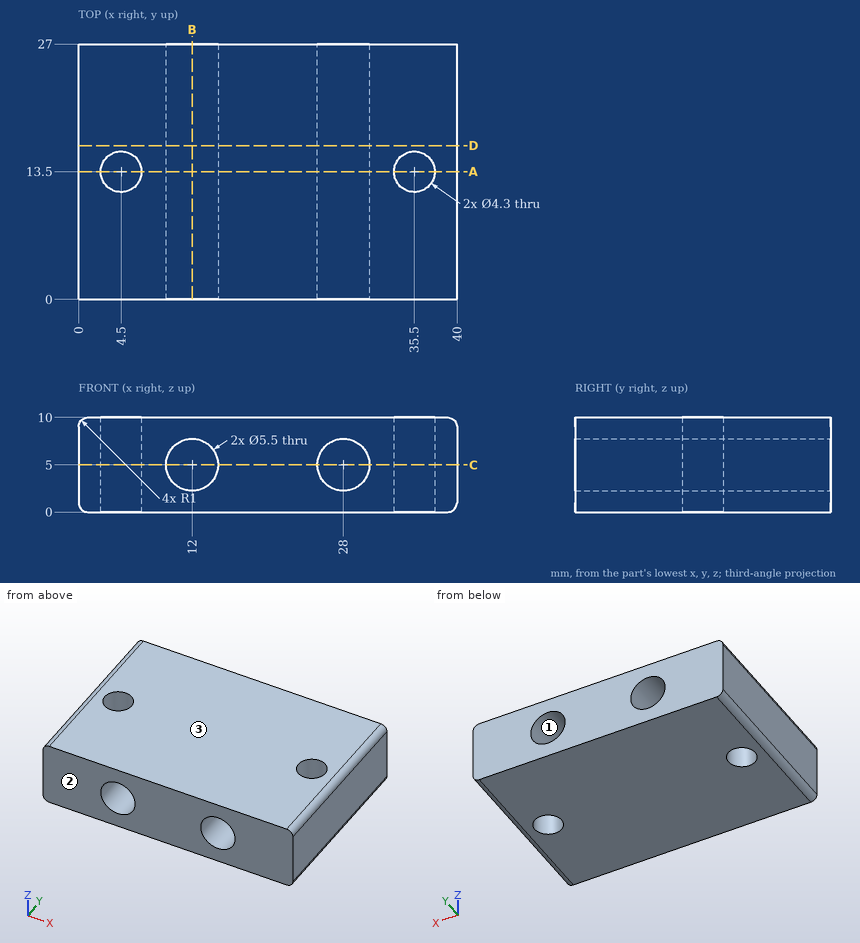
The figure shows three views and two pictorial views of one solid part (mm, origin at its lowest corner). Answer the questions. Coordinates: 2 decimals unless noted, no trailing zeros. Loops run counter-clockwise (first coordinate to the right, second up) from the corner with the lowest first, then second, coordinate; pieces in that order, holes last. Notation, with made-up numbers: M 83,24.5 L 87,24.5 A28 ccw 87,46.5 Z; hole C 84.5,44.5 d7. An arc over 180 degrees is marked long. Use CSV: the item, a comma, the result in double quotes. Start each with the question number.
(1) Find section C-C, the plane z = 5. Give the vertices of the cut face in (x, y).
(2) For a pull along Z with two mould halves and no side action, classify the marked faces 1, 2 and 3 as +Z half, -Z half, draft (parallel to the pull), parting line (faces both ways), or undercut.
(3) Find section A-A, the plane y = 13.5. Give the vertices of the cut face in (x, z).
(4) Find section B-B, the plane x = 12. Give the vertices of the cut face in (y, z), then the cut area to 4 significant figures.
(5) Consider line 1 (X direction, y = 6.75, z = 5); line 2 (Z direction, x = 28, y = 12.5); line 3 (Y direction, x = 4.5, z = 6.5). Determine where each line is inside the solid, lowest interval first.
(6) Find section D-D, the plane y = 16.25. Give the vertices of the cut face in (x, z).
Recorded:
1,outline,"M 0,0 L 9.25,0 L 9.25,27 L 0,27 Z; M 14.75,0 L 25.25,0 L 25.25,27 L 14.75,27 Z; M 30.75,0 L 40,0 L 40,27 L 30.75,27 Z; hole C 4.5,13.5 d4.3; hole C 35.5,13.5 d4.3"
2,face 1,"undercut"
2,face 2,"draft"
2,face 3,"+Z half"
3,outline,"M 0,1 A1 ccw 1,0 L 2.35,0 L 2.35,10 L 1,10 A1 ccw 0,9 Z; M 6.65,0 L 33.35,0 L 33.35,10 L 6.65,10 Z; M 37.65,0 L 39,0 A1 ccw 40,1 L 40,9 A1 ccw 39,10 L 37.65,10 Z; hole C 12,5 d5.5; hole C 28,5 d5.5"
4,outline,"M 0,0 L 27,0 L 27,2.25 L 0,2.25 Z; M 0,7.75 L 27,7.75 L 27,10 L 0,10 Z"
4,area,"121.5 mm^2"
5,line 1,"x = 0 to 9.25, 14.75 to 25.25, 30.75 to 40"
5,line 2,"z = 0 to 2.25, 7.75 to 10"
5,line 3,"y = 0 to 11.35, 15.65 to 27"
6,outline,"M 0,1 A1 ccw 1,0 L 39,0 A1 ccw 40,1 L 40,9 A1 ccw 39,10 L 1,10 A1 ccw 0,9 Z; hole C 12,5 d5.5; hole C 28,5 d5.5"
